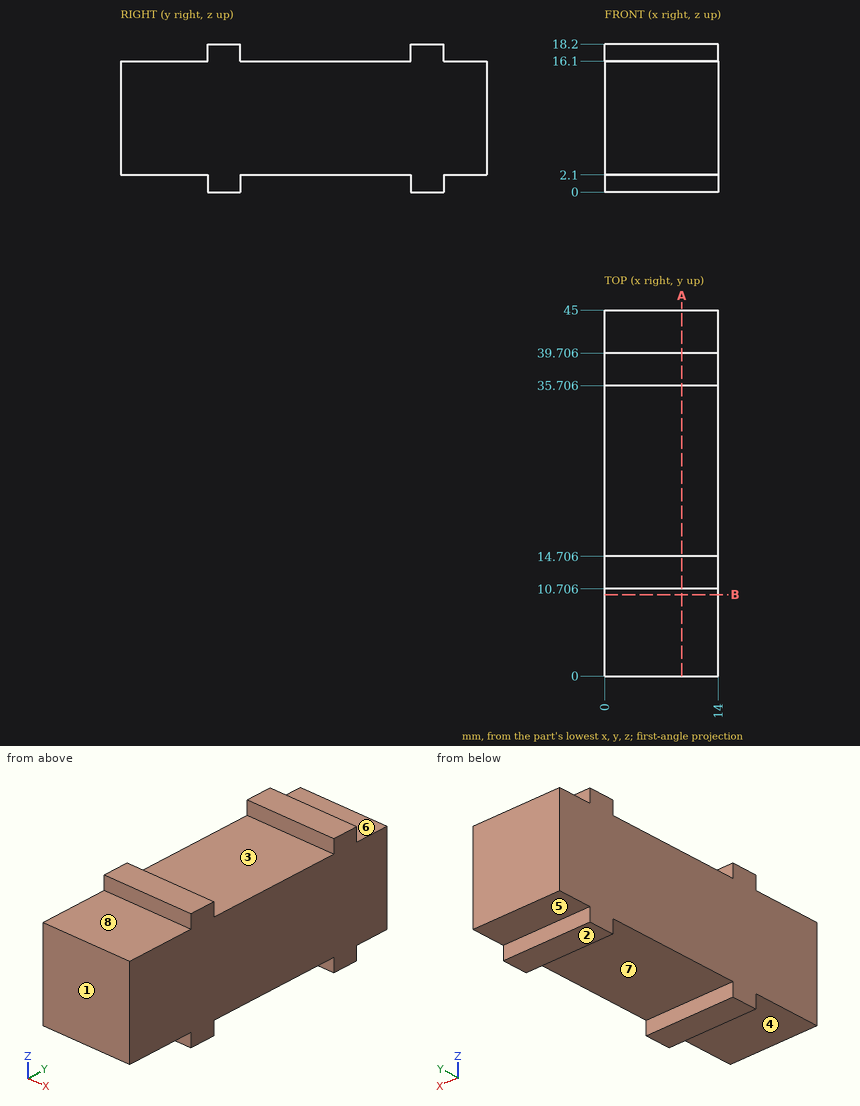
Source: three-view drawing plus pictorial views. Frame: mm from the lowest corner of the part. A direction names the side the tool comes from. Round coordinates to 2 decimals unless told otherwise and drop trailing zeros. Order: outer loops, then holes, each group sorted by start corner. A loop starts at its lowest first (then second) coordinate and runs counter-clockwise, first axis right, second up. Notation, with made-up numbers: (30, 21.25) -> (80, 21.25) arc R19 cw to (80, 31.25) -> close; hole circle Ø9 at (29, -37.5). An arc over 180 degrees is marked (long way). Use CSV: the item, a comma, the result in double quotes. Start each with the question number.
1) Draft query along Y for the marked faces 1, 2 and 3. Return one class per face: +Y half, -Y half, draft (parallel to the pull), parting line (faces both ways), or undercut.
2) Section B-B (y = 10). Return the cut outline in (x, z), and give its area (3 significant figures).
3) First-contact query: pin 1 Ø1.6 at (x, y) = (6.5, 42) entering from +Z; pin 2 Ø3 at (x, y) = (8, 4.5) entering from -Z; pin 3 Ø1.7 at (x, z) = (8, 17.5) entering from -Y. Flat tips, straight axial feed; report the tip coordinate or a pass-through.
4) Set-up query: the marked faces 4, 5, 6, 7 and 8. Return all of +Z, -Z, +X, -X, +Y, -Y with unobstructed straight access to the full face (end or side cutting, diameter ignored); none if empty.
5) Material intervals for line 1 along Y through (x, z) = (5, 17.75); line 2 along Z through (x, y) = (2, 35), sorted ascending. Write a range as from..to.
6) Section A-A (x = 9.5). Return the cut outline in (y, z), and give its area (3 significant figures).
Returned:
1,face 1,"-Y half"
1,face 2,"draft"
1,face 3,"undercut"
2,outline,"(0, 2.1) -> (14, 2.1) -> (14, 16.1) -> (0, 16.1) -> close"
2,area,"196 mm²"
3,pin 1,"stops at z = 16.1"
3,pin 2,"stops at z = 2.1"
3,pin 3,"stops at y = 10.71"
4,face 4,"-Z, +X, -X, -Y"
4,face 5,"-Z, +X, -X, +Y"
4,face 6,"+Z, +X, -X, +Y"
4,face 7,"-Z, +X, -X"
4,face 8,"+Z, +X, -X, -Y"
5,line 1,"y = 10.71..14.71, 35.71..39.71"
5,line 2,"z = 2.1..16.1"
6,outline,"(0, 2.1) -> (10.71, 2.1) -> (10.71, 0) -> (14.71, 0) -> (14.71, 2.1) -> (35.71, 2.1) -> (35.71, 0) -> (39.71, 0) -> (39.71, 2.1) -> (45, 2.1) -> (45, 16.1) -> (39.71, 16.1) -> (39.71, 18.2) -> (35.71, 18.2) -> (35.71, 16.1) -> (14.71, 16.1) -> (14.71, 18.2) -> (10.71, 18.2) -> (10.71, 16.1) -> (0, 16.1) -> close"
6,area,"664 mm²"
